Can you work these out from the model? Positions are in its coordinate system, mm. Give positions to 0.01 mm unless a question says otherwise; leave off trailing zeros. Loops run counter-clockwise (first coordinate to the right, second up) from the corner with the lowest first, then second, coordinate; pieces in that order, holes last. Notation, with made-up numbers: M -26.5,70.5 L 4.5,70.5 A24 cw 4.5,86.5 Z; hole C -14,-27.75 d7. An arc over 180 degrees is marked long. Answer as a JSON object with one key per item and string values.
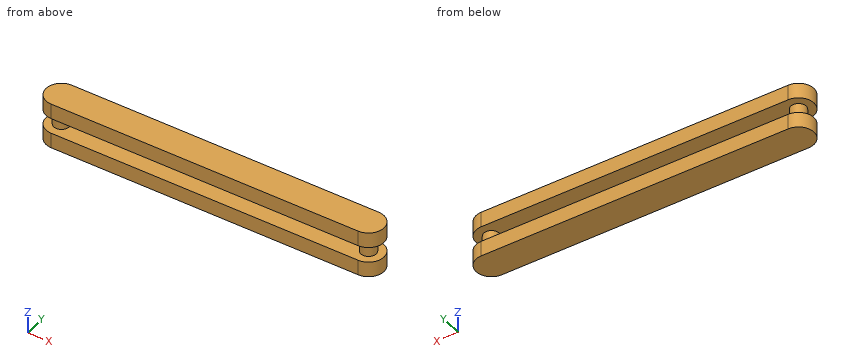
```python
from build123d import *

# Parameters (mm, degrees)
EXTRUDE001_DEPTH = 5
ARRAY_Z_COUNT    = 2
ARRAY_Z_PITCH    = 10
SKETCH002_R      = 2.5
EXTRUDE002_DEPTH = 5


with BuildPart() as array:
    # Sketch001 → Extrude001 (new body)
    with BuildSketch(Plane.XY.offset(-5)):
        with BuildLine():
            ThreePointArc((100, -5), (105, 0), (100, 5))
            Line((0, 5), (100, 5))
            ThreePointArc((0, 5), (-5, 0), (0, -5))
            Line((100, -5), (0, -5))
        make_face()
    extrude(amount=EXTRUDE001_DEPTH)

    # Array Z: Array ×2


with BuildPart() as array_1:
    add(array.part)
    with Locations(*[(0, 0, i * ARRAY_Z_PITCH) for i in range(1, ARRAY_Z_COUNT)]):
        add(array.part)


with BuildPart() as fusion:
    # Sketch002 (on Face6 of Array) → Extrude002 (new body)
    with BuildSketch(Plane.XY):
        Circle(SKETCH002_R)
        with Locations((100, 0)):
            Circle(SKETCH002_R)
    extrude(amount=EXTRUDE002_DEPTH)

    # Fusion: union Array
    add(array_1.part)


solid = fusion.part
```
1) Suppose I cut it at D-D, the plane z = 1.5. Write out the boundary of the cut face in (x, y).
Answer list:
{"outline": "C 0,0 d5; C 100,0 d5"}
2) Suppose I cut it at B-B, the plane y = 0. Write out the boundary of the cut face in (x, z), and give its area (3 significant figures).
Answer list:
{"outline": "M -5,-5 L 105,-5 L 105,0 L 102.5,0 L 102.5,5 L 105,5 L 105,10 L -5,10 L -5,5 L -2.5,5 L -2.5,0 L -5,0 Z; hole M 2.5,0 L 97.5,0 L 97.5,5 L 2.5,5 Z", "area": "1,150 mm^2"}
3) Suppose I cut it at A-A, the plane y = 4. Write out the boundary of the cut face in (x, z), and give its area (3 significant figures).
Answer list:
{"outline": "M -3,-5 L 103,-5 L 103,0 L -3,0 Z; M -3,5 L 103,5 L 103,10 L -3,10 Z", "area": "1,060 mm^2"}
4) Please list where these lines run through material, in increasing order: line 1 along Z through (x, y) = (16.5, -1.5); line 2 along X through (y, z) = (-0.25, 2); line 3 along X through (y, z) = (4.25, 5.5). Write a range as from..to.
Answer list:
{"line 1": "-5..0, 5..10", "line 2": "-2.49..2.49, 97.51..102.49", "line 3": "-2.63..102.63"}
5) Suppose I cut it at C-C, the plane x = 74. Write out the boundary of the cut face in (y, z), and give its area (3 significant figures).
Answer list:
{"outline": "M -5,-5 L 5,-5 L 5,0 L -5,0 Z; M -5,5 L 5,5 L 5,10 L -5,10 Z", "area": "100 mm^2"}
